Design review of the part built by this model. Coordinates are the model's own, in mm. Face numbers are marked on the shaded views. A direction names the side the tool comes from. Coordinates: 2 decimals unless noted, no trailing zeros. Loops run counter-clockwise (first coordinate to the right, second up) from the corner with the lowest first, then second, coordinate; pieces in that order, holes last. Notation, with made-up numbers: M 50,49 L 82,49 A15 cw 82,53 Z; hole C -6,47.25 d3. An arc over 180 degrees is marked long. Answer as a JSON object with one key per item and string values. Group by question number.
1. To check wall thickness, follow probe 1 along X at (y, z) = (122.5, 37); probe 2 along Y at (x, z) = (-82.5, 60); probe 3 along X at (y, z) = (40, 50). State the ranges of each line that lie inside material, in increasing order.
2. Consider section A-A (x = -47). State the section outline as (y, z) points.
3. Consider section B-B (x = -83). State the section outline as (y, z) points, then the cut area to 3 significant figures.
4. Draft analysis for pull direction X (two halves, no side actions). For the marked faces 3, 4, 5 and 6, state which applies: +X half, -X half, draft (parallel to the pull), parting line (faces both ways), or undercut.
5. Machinability: for the marked faces 1 and 2, which of the approach directions +Z, -Z, +X, -X, +Y, -Y give a long, thin tool a straight path to every point of the face, cutting with its end or side? Answer none if there is none.
6. Insertion check: pin 1 (1 mm diameter, centred on y = 128.5, z = 14.5, fed in from -X); pin 2 (1.3 mm diameter, centred on x = -117.54, z = 22.94, fed in from +Y); pin 3 (6.5 mm diameter, centred on x = -119.5, z = 48.5, fed in from +Y). Each pin has a flat end and moves straight along its axis. Give the tip position at first contact, or say it passes through.
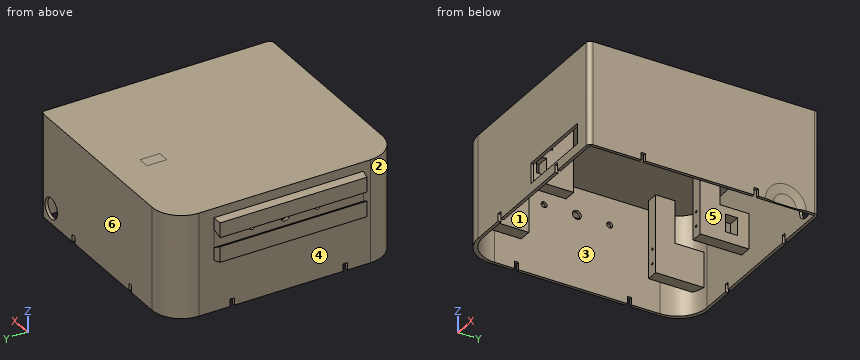
from build123d import *

# Parameters (mm, degrees)
ESQUISSE2_W              = 144.907881123
ESQUISSE2_H              = 156.330521118
BOSS_EXTRU_1_DEPTH       = 70
COQUE1_T                 = -2
ESQUISSE14_W             = 28.733729995
ESQUISSE14_H             = 101.576382864
BOSS_EXTRU_7_DEPTH       = 5.5
BOSS_EXTRU_7_TAPER       = 10
ENL_V_MAT_EXTRU_5_DEPTH  = 137.5
ESQUISSE16_R             = 3
ENL_V_MAT_EXTRU_6_DEPTH  = 3
ESQUISSE17_W             = 8
ESQUISSE17_H             = 24
BOSS_EXTRU_8_DEPTH       = 33
ESQUISSE18_W             = 12.041056231
ESQUISSE18_H             = 8.214509438
ENL_V_MAT_EXTRU_7_DEPTH  = 9
ESQUISSE19_R             = 0.8
ENL_V_MAT_EXTRU_8_DEPTH  = 5
ESQUISSE20_W             = 8.5
ESQUISSE20_H             = 24
BOSS_EXTRU_9_DEPTH       = 33
ESQUISSE22_W             = 11.894232579
ESQUISSE22_H             = 6.744261383
ENL_V_MAT_EXTRU_9_DEPTH  = 10
ESQUISSE25_W             = 8
ESQUISSE25_H             = 13.466046283
BOSS_EXTRU_10_DEPTH      = 30.549003
ESQUISSE26_W             = 8
ESQUISSE26_H             = 13.295181457
BOSS_EXTRU_11_DEPTH      = 30
ESQUISSE27_W             = 8.5
ESQUISSE27_H             = 13.691611871
BOSS_EXTRU_12_DEPTH      = 30
ESQUISSE28_W             = 8.5
ESQUISSE28_H             = 14.379576359
BOSS_EXTRU_14_DEPTH      = 29
ESQUISSE29_R             = 7
ENL_V_MAT_EXTRU_11_DEPTH = 5
ESQUISSE30_W             = 52.718186521
ESQUISSE30_H             = 13.817926224
ENL_V_MAT_EXTRU_12_DEPTH = 5
CONG_4_R                 = 20
CONG_5_R                 = 3
ENL_V_MAT_EXTRU_13_DEPTH = 1
CONG_6_R                 = 20
ESQUISSE21_R             = 0.8
ENL_V_MAT_EXTRU_14_DEPTH = 7
ESQUISSE34_W             = 2
ESQUISSE34_H             = 3
ESQUISSE34_W_2           = 3
ESQUISSE34_H_2           = 2
ENL_V_MAT_EXTRU_15_DEPTH = 5


with BuildPart() as part:
    # Esquisse2 → Boss.-Extru.1 (new body)
    with BuildSketch(Plane.XY):
        with Locations((-60.376721844, 72.874764276)):
            Rectangle(ESQUISSE2_W, ESQUISSE2_H)
    extrude(amount=BOSS_EXTRU_1_DEPTH)

    # Coque1
    coque1_openings = [part.faces().sort_by_distance(p)[0] for p in [
        (-60.376721844, 72.874764276, 0),
    ]]
    offset(amount=COQUE1_T, openings=coque1_openings, kind=Kind.INTERSECTION)

    # Esquisse14 → Boss.-Extru.7 (add)
    with BuildSketch(Plane.ZY.offset(132.830662405)):
        with Locations((49.34125564, 70.231172893)):
            Rectangle(ESQUISSE14_W, ESQUISSE14_H)
    extrude(amount=BOSS_EXTRU_7_DEPTH, taper=BOSS_EXTRU_7_TAPER)

    # Troue matien spirobs → Enlèv. mat.-Extru.5 (cut)
    # profile 1 of 2: a face of its own
    with BuildSketch(Plane(origin=(0, 0, 0), x_dir=(1, 0, 0), z_dir=(0, 1, 0))):
        Polygon((-132.851084635, -55.85540738), (-138.851094768, -52.391307109), (-138.851094768, -46.813956352), (-132.851084635, -43.34985608), align=None)
        Polygon((-133.351084635, -54.989382875), (-138.351094768, -52.102631674), (-138.351094768, -47.102631786), (-133.351084635, -44.215880585), align=None, mode=Mode.SUBTRACT)
    # profile 2 of 2: a face of its own
    with BuildSketch(Plane(origin=(0, 0, 0), x_dir=(1, 0, 0), z_dir=(0, 1, 0))):
        Polygon((-138.351094768, -52.102631674), (-138.351094768, -47.102631786), (-133.351084635, -44.215880585), (-133.351084635, -54.989382875), align=None)
    extrude(amount=ENL_V_MAT_EXTRU_5_DEPTH, mode=Mode.SUBTRACT)

    # Esquisse16 → Enlèv. mat.-Extru.6 (cut)
    with BuildSketch(Plane.ZY.offset(132.851084635)):
        with BuildLine():
            ThreePointArc((51.60263173, 94.988881377), (51.016845292, 96.403094939), (49.60263173, 96.988881377))
            Line((49.60263173, 96.988881377), (49.60263173, 92.988881377))
            ThreePointArc((49.60263173, 92.988881377), (51.016845292, 93.574667814), (51.60263173, 94.988881377))
        make_face()
        with BuildLine():
            Line((49.60263173, 92.988881377), (49.60263173, 96.988881377))
            ThreePointArc((49.60263173, 96.988881377), (47.60263173, 94.988881377), (49.60263173, 92.988881377))
        make_face()
        with BuildLine():
            ThreePointArc((51.60263173, 50.488881377), (51.016845292, 51.903094939), (49.60263173, 52.488881377))
            Line((49.60263173, 52.488881377), (49.60263173, 48.488881377))
            ThreePointArc((49.60263173, 48.488881377), (51.016845292, 49.074667814), (51.60263173, 50.488881377))
        make_face()
        with BuildLine():
            Line((49.60263173, 48.488881377), (49.60263173, 52.488881377))
            ThreePointArc((49.60263173, 52.488881377), (47.60263173, 50.488881377), (49.60263173, 48.488881377))
        make_face()
        with Locations((49.60263173, 72.738881377)):
            Circle(ESQUISSE16_R)
    extrude(amount=-ENL_V_MAT_EXTRU_6_DEPTH, mode=Mode.SUBTRACT)

    # Esquisse17 → Boss.-Extru.8 (add)
    with BuildSketch(Plane.XZ.offset(-149.040024835)):
        with Locations((-67.645104732, 27.450996733)):
            Rectangle(ESQUISSE17_W, ESQUISSE17_H)
        with Locations((-117.942168048, 27.160873918)):
            Rectangle(ESQUISSE17_W, ESQUISSE17_H)
    extrude(amount=BOSS_EXTRU_8_DEPTH)

    # Esquisse18 → Enlèv. mat.-Extru.7 (cut)
    with BuildSketch(Plane(origin=(-63.645104732, 0, 0), x_dir=(0, 0, -1), z_dir=(1, 0, 0))):
        with Locations((-28.237409826, 137.403900729)):
            Rectangle(ESQUISSE18_W, ESQUISSE18_H)
    extrude(amount=-ENL_V_MAT_EXTRU_7_DEPTH, mode=Mode.SUBTRACT)

    # Esquisse19 → Enlèv. mat.-Extru.8 (cut)
    with BuildSketch(Plane.XZ.offset(-116.040024835)):
        with Locations(Location((-68.110177619, 23.053024635, 0), (0, 0, 270))):
            Circle(ESQUISSE19_R)
        with Locations(Location((-68.110177619, 32.817579673, 0), (0, 0, 270))):
            Circle(ESQUISSE19_R)
        with Locations(Location((-117.542963794, 32.93870849, 0), (0, 0, 270))):
            Circle(ESQUISSE19_R)
        with Locations(Location((-117.542963794, 22.93870849, 0), (0, 0, 270))):
            Circle(ESQUISSE19_R)
    extrude(amount=-ENL_V_MAT_EXTRU_8_DEPTH, mode=Mode.SUBTRACT)

    # Esquisse20 → Boss.-Extru.9 (add)
    with BuildSketch(Plane(origin=(0, -3.290496283, 0), x_dir=(1, 0, 0), z_dir=(0, 1, 0))):
        with Locations((-117.838572927, -27.374102793)):
            Rectangle(ESQUISSE20_W, ESQUISSE20_H)
        with Locations((-67.264692574, -28.393869792)):
            Rectangle(ESQUISSE20_W, ESQUISSE20_H)
    extrude(amount=BOSS_EXTRU_9_DEPTH)

    # Esquisse22 → Enlèv. mat.-Extru.9 (cut)
    with BuildSketch(Plane(origin=(-63.014692574, 0, 0), x_dir=(0, 0, -1), z_dir=(1, 0, 0))):
        with Locations((-27.890614159, 7.930587585)):
            Rectangle(ESQUISSE22_W, ESQUISSE22_H)
    extrude(amount=-ENL_V_MAT_EXTRU_9_DEPTH, mode=Mode.SUBTRACT)

    # Esquisse25 → Boss.-Extru.10 (add)
    with BuildSketch(Plane.XY.offset(39.450996733)):
        with Locations((-67.645104732, 122.773047977)):
            Rectangle(ESQUISSE25_W, ESQUISSE25_H)
    extrude(amount=BOSS_EXTRU_10_DEPTH)

    # Esquisse26 → Boss.-Extru.11 (add)
    with BuildSketch(Plane.XY.offset(39.160873918)):
        with Locations((-117.942168048, 122.687615564)):
            Rectangle(ESQUISSE26_W, ESQUISSE26_H)
    extrude(amount=BOSS_EXTRU_11_DEPTH)

    # Esquisse27 → Boss.-Extru.12 (add)
    with BuildSketch(Plane.XY.offset(39.374102793)):
        with Locations((-117.838572927, 22.863697782)):
            Rectangle(ESQUISSE27_W, ESQUISSE27_H)
    extrude(amount=BOSS_EXTRU_12_DEPTH)

    # Esquisse28 → Boss.-Extru.14 (add)
    with BuildSketch(Plane.XY.offset(40.393869792)):
        with Locations((-67.264692574, 22.519715538)):
            Rectangle(ESQUISSE28_W, ESQUISSE28_H)
    extrude(amount=BOSS_EXTRU_14_DEPTH)

    # Esquisse29 → Enlèv. mat.-Extru.11 (cut)
    with BuildSketch(Plane(origin=(0, 151.040024835, 0), x_dir=(1, 0, 0), z_dir=(0, 1, 0))):
        with Locations(Location((0.637722391, -10.29069879, 0), (0, 0, 270))):
            Circle(ESQUISSE29_R)
    extrude(amount=-ENL_V_MAT_EXTRU_11_DEPTH, mode=Mode.SUBTRACT)

    # Esquisse30 → Enlèv. mat.-Extru.12 (cut)
    with BuildSketch(Plane.XZ.offset(5.290496283)):
        with Locations((-26.862211313, 13.280210157)):
            Rectangle(ESQUISSE30_W, ESQUISSE30_H)
    extrude(amount=-ENL_V_MAT_EXTRU_12_DEPTH, mode=Mode.SUBTRACT)

    # Congé4
    # the kernel refuses this fillet: 20 mm, written as the material it adds along each edge
    with BuildSketch(Plane(origin=(-130.830662405, 149.040024835, 0), x_dir=(1, 0, 0), z_dir=(0, 0, 1))) as cong_4_piece_1:
        with BuildLine():
            CenterArc((CONG_4_R, -CONG_4_R), CONG_4_R, 90, 90)
            Line((0, -CONG_4_R), (0, 0))
            Line((0, 0), (CONG_4_R, 0))
        make_face()
    extrude(amount=68)
    with BuildSketch(Plane(origin=(-130.830662405, -3.290496283, 68), x_dir=(0, 1, 0), z_dir=(0, 0, -1))) as cong_4_piece_2:
        with BuildLine():
            CenterArc((CONG_4_R, CONG_4_R), CONG_4_R, 180, 90)
            Line((0, CONG_4_R), (0, 0))
            Line((0, 0), (CONG_4_R, 0))
        make_face()
    extrude(amount=68)
    # the kernel refuses this fillet: 20 mm, written as the material it takes off along each edge
    with BuildSketch(Plane(origin=(-132.830662405, -5.290496283, -50), x_dir=(0, 1, 0), z_dir=(0, 0, 1)), Plane(origin=(-132.830662405, 151.040024835, -50), x_dir=(1, 0, 0), z_dir=(0, 0, 1))) as cong_4_2_piece_1:
        with BuildLine():
            CenterArc((CONG_4_R, -CONG_4_R), CONG_4_R, 90, 90)
            Line((0, -CONG_4_R), (0, 0))
            Line((0, 0), (CONG_4_R, 0))
        make_face()
    extrude(amount=170, mode=Mode.SUBTRACT)

    # Congé5
    cong_5_edges = [part.edges().sort_by_distance(p)[0] for p in [
        (12.077218718, -5.290496283, 35),
        (12.077218718, 151.040024835, 35),
    ]]
    fillet(cong_5_edges, radius=CONG_5_R)

    # Esquisse31 → Enlèv. mat.-Extru.13 (cut)
    with BuildSketch(Plane(origin=(12.077218718, 0, 0), x_dir=(0, 0, -1), z_dir=(1, 0, 0))):
        with BuildLine():
            Line((0, 120.991434469), (0, 136.191208624))
            ThreePointArc((0, 136.191208624), (-7.599887078, 128.591321546), (0, 120.991434469))
        make_face()
    extrude(amount=-ENL_V_MAT_EXTRU_13_DEPTH, mode=Mode.SUBTRACT)

    # Congé6
    # the kernel refuses this fillet: 20 mm, written as the material it takes off along each edge
    with BuildSketch(Plane(origin=(12.077218718, 128.591321546, 0), x_dir=(0, 0.003141587485881077, -0.9999950652018582), z_dir=(0, -0.9999950652018582, -0.003141587485881077))) as cong_6_piece_1:
        with BuildLine():
            CenterArc((13.844885076, -20), CONG_6_R, 90, 18.194872339)
            Line((7.599887078, -1), (7.474987118, -0.62))
            ThreePointArc((7.474987118, -0.62), (7.199887078, -0.5), (7.199887078, 0))
            Line((7.199887078, 0), (7.599887078, 0.4))
            Line((7.599887078, 0.4), (13.844885076, 0.4))
            Line((13.844885076, 0.4), (13.844885076, 0))
        make_face()
    revolve(axis=Axis((12.077218718, 128.591321546, 0), (1, 0, 0)), revolution_arc=359.64, mode=Mode.SUBTRACT)

    # Esquisse21 → Enlèv. mat.-Extru.14 (cut)
    with BuildSketch(Plane(origin=(0, 29.709503717, 0), x_dir=(1, 0, 0), z_dir=(0, 1, 0))):
        with Locations(Location((-68.061939997, -22.535603051, 0), (0, 0, 270))):
            Circle(ESQUISSE21_R)
        with Locations(Location((-68.061939997, -32.603026975, 0), (0, 0, 270))):
            Circle(ESQUISSE21_R)
        with Locations(Location((-117.577847279, -22.535603051, 0), (0, 0, 270))):
            Circle(ESQUISSE21_R)
        with Locations(Location((-117.561939997, -32.372185179, 0), (0, 0, 270))):
            Circle(ESQUISSE21_R)
    extrude(amount=-ENL_V_MAT_EXTRU_14_DEPTH, mode=Mode.SUBTRACT)

    # Esquisse34 → Enlèv. mat.-Extru.15 (cut)
    with BuildSketch(Plane(origin=(0, 0, 0), x_dir=(-1, 0, 0), z_dir=(0, 0, -1))):
        with Locations((131.830662405, 31.752830171)):
            Rectangle(ESQUISSE34_W, ESQUISSE34_H)
        with Locations((131.830662405, 108.450383814)):
            Rectangle(ESQUISSE34_W, ESQUISSE34_H)
        with Locations((-11.077218718, 31.752830171)):
            Rectangle(ESQUISSE34_W, ESQUISSE34_H)
        with Locations((-11.077218718, 108.450383814)):
            Rectangle(ESQUISSE34_W, ESQUISSE34_H)
        with Locations((88.44920315, 150.040024835)):
            Rectangle(ESQUISSE34_W_2, ESQUISSE34_H_2)
        with Locations((24.448737585, 150.040024835)):
            Rectangle(ESQUISSE34_W_2, ESQUISSE34_H_2)
        with Locations((24.448737585, -4.290496283)):
            Rectangle(ESQUISSE34_W_2, ESQUISSE34_H_2)
        with Locations((88.44920315, -4.290496283)):
            Rectangle(ESQUISSE34_W_2, ESQUISSE34_H_2)
    extrude(amount=-ENL_V_MAT_EXTRU_15_DEPTH, mode=Mode.SUBTRACT)


solid = part.part
Findings below:
{
 "1": {"probe 1": "x = -132.83 to -130.83, -121.94 to -113.94, -71.65 to -63.65, 10.08 to 12.08", "probe 2": "y = -5.29 to -3.29, 149.04 to 151.04", "probe 3": "x = -132.85 to -130.83, 10.08 to 12.08"},
 "2": {"outline": "M -5.29,0 L -3.29,0 L -3.29,6.37 L -5.29,6.37 Z; M -5.29,20.19 L -3.29,20.19 L -3.29,68 L 149.04,68 L 149.04,0 L 151.04,0 L 151.04,70 L -5.29,70 Z"},
 "3": {"outline": "M -5.29,0 L -3.29,0 L -3.29,68 L 149.04,68 L 149.04,0 L 151.04,0 L 151.04,70 L -5.29,70 Z", "area": "585 mm^2"},
 "4": {"face 3": "undercut", "face 4": "-X half", "face 5": "undercut", "face 6": "draft"},
 "5": {"face 1": "-Z", "face 2": "+Z, -Z, -X, -Y"},
 "6": {"pin 1": "stops at x = -132.83", "pin 2": "stops at y = 150.62", "pin 3": "stops at y = 150.75"}
}
